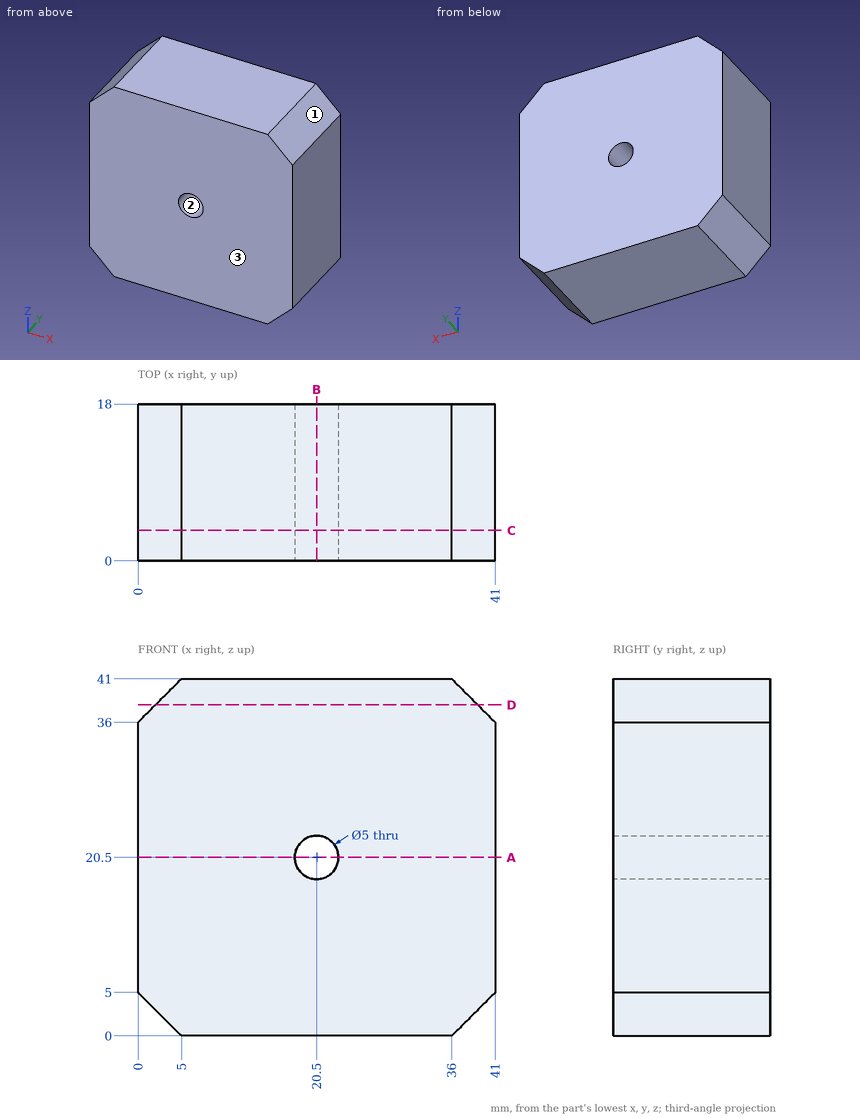
Here's the drawing with two shaded views (mm, measured from the low corner). I have some questions. Give positions to 0.01 mm unless a question says otherwise; leave off trailing zeros. Order: outer loops, then holes, each group sorted by start corner. A loop starts at its lowest first (then second) coordinate and runs counter-clockwise, first axis right, second up. Notation, with made-up numbers: M 76.25,14.5 L 99.25,14.5 A16 cw 99.25,43.5 Z; hole C 82,-7.5 d2. An arc over 180 degrees is marked long. One line per item, written item: value.
1) I want a section at D-D, the plane z = 38. List the corners of the cut face in (x, y) for me.
Answer sheet:
outline: M 2,0 L 39,0 L 39,18 L 2,18 Z
2) We'd pull the mould along X, two halves only. Please class the marked faces 1, 2 and 3: released by +X, released by -X, zero draft, split by the parting line, or undercut.
Answer sheet:
face 1: released by +X
face 2: undercut
face 3: zero draft
3) I want a section at B-B, the plane x = 20.5. List the corners of the cut face in (y, z) for me, plus the area to 3 significant figures.
Answer sheet:
outline: M 0,0 L 18,0 L 18,18 L 0,18 Z; M 0,23 L 18,23 L 18,41 L 0,41 Z
area: 648 mm^2
4) I want a section at C-C, the plane y = 3.5. List the corners of the cut face in (x, z) for me, plus the area to 3 significant figures.
Answer sheet:
outline: M 0,5 L 5,0 L 36,0 L 41,5 L 41,36 L 36,41 L 5,41 L 0,36 Z; hole C 20.5,20.5 d5
area: 1,610 mm^2
5) Please list where these lines run through material, in increasing order: line 1 along Z through (x, y) = (20.5, 9); line 2 along X through (y, z) = (0.5, 22).
Answer sheet:
line 1: z = 0 to 18, 23 to 41
line 2: x = 0 to 18.5, 22.5 to 41
6) I want a section at A-A, the plane z = 20.5. List the corners of the cut face in (x, y) for me, plus the area to 3 significant figures.
Answer sheet:
outline: M 0,0 L 18,0 L 18,18 L 0,18 Z; M 23,0 L 41,0 L 41,18 L 23,18 Z
area: 648 mm^2
